from build123d import *

# Parameters (mm, degrees)
SKETCH1_W           = 50.8
SKETCH1_H           = 50.8
SKETCH1_W_2         = 44.45
SKETCH1_H_2         = 44.45
BOSS_EXTRUDE1_DEPTH = 260.35
SKETCH2_R           = 25.4
CUT_EXTRUDE1_DEPTH  = 51.8
SKETCH3_R           = 3.96875
CUT_EXTRUDE2_DEPTH  = 51.8


with BuildPart() as part:
    # Sketch1 → Boss-Extrude1 (new body)
    with BuildSketch(Plane.XY):
        with Locations((25.4, 25.4)):
            Rectangle(SKETCH1_W, SKETCH1_H)
        with Locations((25.4, 25.4)):
            Rectangle(SKETCH1_W_2, SKETCH1_H_2, mode=Mode.SUBTRACT)
    extrude(amount=BOSS_EXTRUDE1_DEPTH)

    # Sketch2 → Cut-Extrude1 (cut, through all)
    with BuildSketch(Plane(origin=(50.8, 0, 0), x_dir=(0, 0, -1), z_dir=(1, 0, 0))):
        with Locations((-266.7, 25.4)):
            Circle(SKETCH2_R)
    extrude(amount=-CUT_EXTRUDE1_DEPTH, mode=Mode.SUBTRACT)

    # Sketch3 → Cut-Extrude2 (cut, through all)
    with BuildSketch(Plane.XZ):
        with Locations((38.1, 76.735833685)):
            Circle(SKETCH3_R)
        with Locations((12.7, 53.175)):
            Circle(SKETCH3_R)
    extrude(amount=-CUT_EXTRUDE2_DEPTH, mode=Mode.SUBTRACT)


solid = part.part
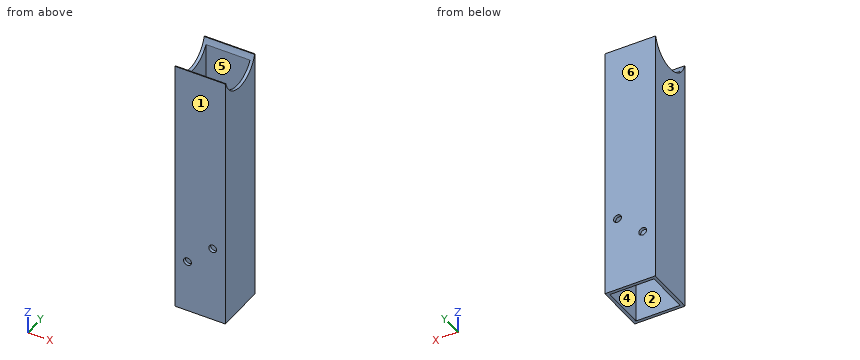
Work out the finished part from the listing and answer in its coordinate system (mm). Face numbers are marked on the shaded views. A direction names the side the tool comes from. Coordinates: 2 decimals unless noted, no trailing zeros. Write each loop counter-clockwise with the first axis right and the second up, starting at its lowest first coordinate (ties: lowest second). Pieces come first, ordered by that corner, then holes.
1. The part is cut by section D-D, the plane z = 138. Write down the section's boundary in (x, y) (3 decimals), and give its area (3 significant figures).
Results list:
outline: (0, 0) - (50.8, 0) - (50.8, 50.8) - (0, 50.8) - close; hole (3.175, 3.175) - (47.625, 3.175) - (47.625, 47.625) - (3.175, 47.625) - close
area: 605 mm2
2. Consider line 1 along Y through (x, z) = (44, 82) (3 decimals); line 2 along Z through (x, y) = (34, 48). Determine where each line is inside the solid, lowest interval first.
Results list:
line 1: y = 0 to 3.175, 47.625 to 50.8
line 2: z = 0 to 255.11
3. A flat-ended cylindrical pin translates along its axis: pin 1 (7 mm diameter, centred on x = 38.1, z = 76.74, fed in from -Y). Find the tip coordinate at first contact, or state that the pin passes through.
Results list:
pin 1: passes through
4. For the marked faces 5 and 6, determine the directions among +Z, -Z, +X, -X, +Y, -Y from which every point of the face is accessible in a straight line to the end or side of a thin tool.
Results list:
face 5: +Z, -Z
face 6: +Z, -Z, +X, -X, +Y
5. For a pull along X with two mould halves and no side action, classify the marked faces 1, 2, 3 and 4 as +X half, -X half, draft (parallel to the pull), parting line (faces both ways), or undercut.
Results list:
face 1: draft
face 2: undercut
face 3: -X half
face 4: undercut
6. The part is cut by section A-A, the plane x = 12.7. Write down the section's boundary in (y, z) (3 decimals).
Results list:
outline: (0, 0) - (3.175, 0) - (3.175, 49.206) - (0, 49.206) - close; (0, 57.144) - (3.175, 57.144) - (3.175, 254.403) arc R25.4 cw to (0.807, 260.35) - (0, 260.35) - close; (47.625, 0) - (50.8, 0) - (50.8, 49.206) - (47.625, 49.206) - close; (47.625, 57.144) - (50.8, 57.144) - (50.8, 260.35) - (49.993, 260.35) arc R25.4 cw to (47.625, 254.403) - close
7. The part is cut by section C-C, the plane x = 30. Write down the section's boundary in (y, z) (3 decimals), and give its area (3 significant figures).
Results list:
outline: (0, 0) - (3.175, 0) - (3.175, 254.403) arc R25.4 cw to (0.807, 260.35) - (0, 260.35) - close; (47.625, 0) - (50.8, 0) - (50.8, 260.35) - (49.993, 260.35) arc R25.4 cw to (47.625, 254.403) - close
area: 1,640 mm2
8. The part is cut by section B-B, the plane y = 19. Write down the section's boundary in (x, z) (3 decimals).
Results list:
outline: (0, 0) - (3.175, 0) - (3.175, 242.12) - (0, 242.12) - close; (47.625, 0) - (50.8, 0) - (50.8, 242.12) - (47.625, 242.12) - close
